```python
from build123d import *

# Parameters (mm, degrees)
BOSS_EXTRUDE2_DEPTH                         = 55
BOSS_EXTRUDE4_DEPTH                         = 20
CUT_EXTRUDE4_DEPTH                          = 78.580603246
CUT_EXTRUDE4_DEPTH_BACK                     = 78.580603246
SKETCH7_R                                   = 4.25
CUT_EXTRUDE5_REACH                          = 79.581
CUT_EXTRUDE5_END_RADIUS                     = 4.25
SKETCH8_R                                   = 2.25
CUT_EXTRUDE6_DEPTH                          = 4
SKETCH2_5_R                                 = 10
CUT_EXTRUDE7_DEPTH                          = 50
FILLET1_R                                   = 4
FILLET3_R                                   = 5
CBORE_FOR_M4_CHEESE_HEAD_SCREW1_D           = 4.5
CBORE_FOR_M4_CHEESE_HEAD_SCREW1_CBORE_D     = 8
CBORE_FOR_M4_CHEESE_HEAD_SCREW1_CBORE_DEPTH = 2.6
CUT_EXTRUDE8_DEPTH                          = 1


with BuildPart() as part:
    # Sketch2 → Boss-Extrude2 (new body)
    with BuildSketch(Plane.XY):
        with BuildLine():
            Line((12.990381057, -7.5), (12.990381057, 7.5))
            ThreePointArc((12.990381057, 7.5), (0, 15), (-12.990381057, 7.5))
            Line((-12.990381057, 7.5), (-12.990381057, -7.5))
            ThreePointArc((-12.990381057, -7.5), (0, -15), (12.990381057, -7.5))
        make_face()
    extrude(amount=-BOSS_EXTRUDE2_DEPTH)

    # Sketch6 → Boss-Extrude4 (add)
    with BuildSketch(Plane(origin=(0, 0, -55), x_dir=(-1, 0, 0), z_dir=(0, 0, -1))):
        with BuildLine():
            ThreePointArc((9.270248109, 3.75), (0, 10), (-9.270248109, 3.75))
            Line((-9.270248109, 3.75), (-9.270248109, -3.75))
            ThreePointArc((-9.270248109, -3.75), (0, -10), (9.270248109, -3.75))
            Line((9.270248109, -3.75), (9.270248109, 3.75))
        make_face()
    extrude(amount=BOSS_EXTRUDE4_DEPTH)

    # Sketch7 → Cut-Extrude4 (cut, two sides: drawn at the far end of the back side and taken through both)
    with BuildSketch(Plane(origin=(0, 0, 0), x_dir=(0, 0, -1), z_dir=(1, 0, 0)).offset(-CUT_EXTRUDE4_DEPTH_BACK)):
        with Locations(Location((65, 0, 0), (0, 0, 298.072486936))):
            Circle(SKETCH7_R)
    extrude(amount=CUT_EXTRUDE4_DEPTH + CUT_EXTRUDE4_DEPTH_BACK, mode=Mode.SUBTRACT)

    # Cut-Extrude5: up to this cylinder (the profile starts outside it)
    cut_extrude5_end = Plane(origin=(0, 0, -65), z_dir=(1, 0, 0)) * Cylinder(CUT_EXTRUDE5_END_RADIUS, 168.662, mode=Mode.PRIVATE)
    # Sketch8 → Cut-Extrude5 (cut, up to the surface)
    with BuildSketch(Plane(origin=(0, 0, -75), x_dir=(-1, 0, 0), z_dir=(0, 0, -1)), mode=Mode.PRIVATE) as cut_extrude5_sk1:
        Circle(SKETCH8_R)
    cut_extrude5_tool1 = extrude(cut_extrude5_sk1.sketch, amount=-CUT_EXTRUDE5_REACH, mode=Mode.PRIVATE) - cut_extrude5_end
    add(cut_extrude5_tool1.solids().sort_by_distance((0, 0, -75))[0], mode=Mode.SUBTRACT)

    # Sketch8<3> → Cut-Extrude6 (cut)
    with BuildSketch(Plane(origin=(0, 0, -75), x_dir=(-1, 0, 0), z_dir=(0, 0, -1))):
        Polygon((3.7, -2.136195996), (3.7, 2.136195996), (0, 4.272391992), (-3.7, 2.136195996), (-3.7, -2.136195996), (0, -4.272391992), align=None)
    extrude(amount=-CUT_EXTRUDE6_DEPTH, mode=Mode.SUBTRACT)

    # Sketch2<5> → Cut-Extrude7 (cut)
    with BuildSketch(Plane.XY):
        Circle(SKETCH2_5_R)
    extrude(amount=-CUT_EXTRUDE7_DEPTH, mode=Mode.SUBTRACT)

    # Fillet1
    # the kernel refuses this fillet: 4 mm, written as the material it takes off along each edge
    with BuildSketch(Plane(origin=(0, 0, -55), x_dir=(-0.9897152245182474, 0.1430516492627579, 0), z_dir=(0.1430516492627579, 0.9897152245182474, 0))) as fillet1_piece_1:
        with BuildLine():
            CenterArc((15 - FILLET1_R, FILLET1_R), FILLET1_R, 270, 90)
            Line((15 - FILLET1_R, 0), (15, 0))
            Line((15, 0), (15, FILLET1_R))
        make_face()
    revolve(axis=Axis((0, 0, -55), (0, 0, 1)), revolution_arc=196.448941493, mode=Mode.SUBTRACT)
    with BuildSketch(Plane(origin=(0, 0, -55), x_dir=(0.9897152245182473, -0.14305164926275812, 0), z_dir=(-0.14305164926275812, -0.9897152245182473, 0))) as fillet1_piece_2:
        with BuildLine():
            CenterArc((15 - FILLET1_R, FILLET1_R), FILLET1_R, 270, 90)
            Line((15 - FILLET1_R, 0), (15, 0))
            Line((15, 0), (15, FILLET1_R))
        make_face()
    revolve(axis=Axis((0, 0, -55), (0, 0, 1)), revolution_arc=196.448941493, mode=Mode.SUBTRACT)

    # Fillet3
    # the kernel refuses this fillet: 5 mm, written as the material it takes off along each edge
    with BuildSketch(Plane(origin=(0, 0, -75), x_dir=(-0.647307646342804, -0.7622288442365189, 0), z_dir=(0.7622288442365189, -0.647307646342804, 0))) as fillet3_piece_1:
        with BuildLine():
            CenterArc((10 - FILLET3_R, -FILLET3_R), FILLET3_R, 0, 90)
            Line((10, -FILLET3_R), (10, 0))
            Line((10, 0), (10 - FILLET3_R, 0))
        make_face()
    revolve(axis=Axis((0, 0, -75), (0, 0, -1)), revolution_arc=279.32216765, mode=Mode.SUBTRACT)
    with BuildSketch(Plane(origin=(0, 0, -75), x_dir=(0.6473076463428042, 0.7622288442365188, 0), z_dir=(-0.7622288442365188, 0.6473076463428042, 0))) as fillet3_piece_2:
        with BuildLine():
            CenterArc((10 - FILLET3_R, -FILLET3_R), FILLET3_R, 0, 90)
            Line((10, -FILLET3_R), (10, 0))
            Line((10, 0), (10 - FILLET3_R, 0))
        make_face()
    revolve(axis=Axis((0, 0, -75), (0, 0, -1)), revolution_arc=279.32216765, mode=Mode.SUBTRACT)

    # CBORE for M4 Cheese Head Screw1 (through all)
    with Locations(Plane(origin=(12.990381057, 0, 0), x_dir=(0, 0, -1), z_dir=(1, 0, 0))):
        with Locations((20, 0)):
            CounterBoreHole(CBORE_FOR_M4_CHEESE_HEAD_SCREW1_D / 2, CBORE_FOR_M4_CHEESE_HEAD_SCREW1_CBORE_D / 2, CBORE_FOR_M4_CHEESE_HEAD_SCREW1_CBORE_DEPTH)

    # Sketch9 → Cut-Extrude8 (cut)
    with BuildSketch(Plane.ZY.offset(12.990381057)):
        Polygon((-15.669872981, 0), (-17.834936491, 3.75), (-22.165063509, 3.75), (-24.330127019, 0), (-22.165063509, -3.75), (-17.834936491, -3.75), align=None)
    extrude(amount=-CUT_EXTRUDE8_DEPTH, mode=Mode.SUBTRACT)


solid = part.part
```
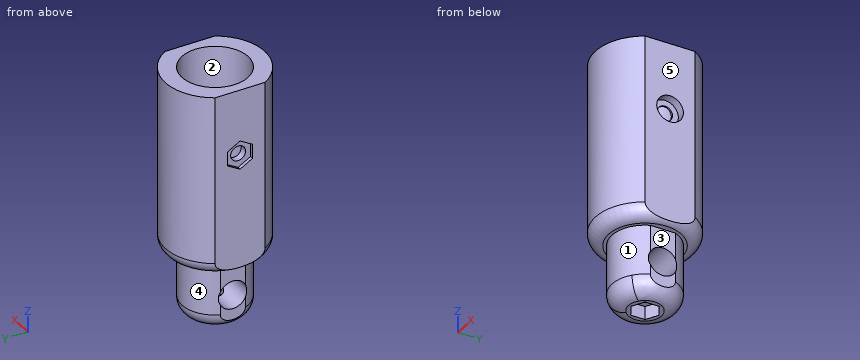
Part model, mm, in its own coordinate system. Face numbers are marked on the shaded views. A direction names the side the tool comes from. Round coordinates to 2 decimals unless told otherwise and drop trailing zeros. Write each loop counter-clockwise with the first axis right and the second up, starting at its lowest first coordinate (ties: lowest second). Pieces come first, ordered by that corner, then holes.
Item 1: Which spindle directions (+Z, -Z, +X, -X, +Y, -Y) get a long thin tool onto all of the face, cutting with end or side? Do the marked faces 4 and 5. Say none if no direction does.
Results:
face 4: -Z, +Y
face 5: +Z, -Z, +X, +Y, -Y
Item 2: Two-plate mould, pull along Y, no slides. Class the marked faces 1, 2 and 3: +Y half, -Y half, draft (parallel to the pull), parting line (faces both ways), or undercut.
Results:
face 1: -Y half
face 2: undercut
face 3: draft
Item 3: Cut at B-B, the plane z = -8.5. Give the cut face in (x, y), plus the area to 3 significant figures.
Results:
outline: (-12.99, -7.5) arc R15 ccw to (12.99, -7.5) - (12.99, 7.5) arc R15 ccw to (-12.99, 7.5) - close; hole circle Ø20 at (0, 0)
area: 352 mm2
Item 4: Probe L1, parallel to X at y = 0, z = -27; L2, parallel to Z at x = 10.1, y = 0; L3, parallel to X at y = 0, z = -69.9. List the from-to ranges inside material, lowest first.
Results:
L1: x = -12.99 to -10, 10 to 12.99
L2: z = -55 to -22.25, -17.75 to 0
L3: x = -9.27 to -2.25, 2.25 to 9.27
Item 5: Cut at A-A, the plane z = -20. Give the cut face in (x, y).
Results:
outline: (-12.99, -7.5) arc R15 ccw to (12.99, -7.5) - (12.99, -4) - (10.39, -4) - (10.39, -2.25) - (9.74, -2.25) arc R10 cw to (-9.74, -2.25) - (-11.99, -2.25) - (-11.99, -3.75) - (-12.99, -3.75) - close; (-12.99, 3.75) - (-11.99, 3.75) - (-11.99, 2.25) - (-9.74, 2.25) arc R10 cw to (9.74, 2.25) - (10.39, 2.25) - (10.39, 4) - (12.99, 4) - (12.99, 7.5) arc R15 ccw to (-12.99, 7.5) - close
Item 6: Cut at C-C, the plane z = -65. Give the cut face in (x, y).
Results:
outline: (-9.05, -4.25) arc R10 ccw to (9.05, -4.25) - close; (-9.05, 4.25) - (9.05, 4.25) arc R10 ccw to start
Item 7: Drop flat-ended pins along their axis: pin 1 Ø3 at (y, z) = (-0.5, -71) entering from -X; pin 2 Ø8 at (x, z) = (5, -42.5) entering from -Y; pin 3 Ø1.2 at (y, z) = (0, -73.5) entering from -X. Give the stop position or say it passes through.
Results:
pin 1: stops at x = -9.27
pin 2: stops at y = -14.97
pin 3: stops at x = -9.07
